from build123d import *

# Parameters (mm, degrees)
SKETCH1_W           = 100
SKETCH1_H           = 58.42
SKETCH1_R           = 2.55
SKETCH1_R_2         = 1.625
SKETCH1_R_3         = 10.5
BOSS_EXTRUDE1_DEPTH = 7.9375
SKETCH2_R           = 4.05
CUT_EXTRUDE1_DEPTH  = 15


with BuildPart() as part:
    # Sketch1 → Boss-Extrude1 (new body)
    with BuildSketch(Plane.XZ.offset(110.068674648)):
        with Locations((45.506748586, 71.609111908)):
            Rectangle(SKETCH1_W, SKETCH1_H)
        with Locations(Location((1.146748586, 95.179111908, 0), (0, 0, 270))):
            Circle(SKETCH1_R, mode=Mode.SUBTRACT)
        with Locations(Location((1.146748586, 48.039111908, 0), (0, 0, 270))):
            Circle(SKETCH1_R, mode=Mode.SUBTRACT)
        with Locations(Location((48.286748586, 48.039111908, 0), (0, 0, 270))):
            Circle(SKETCH1_R, mode=Mode.SUBTRACT)
        with Locations(Location((48.286748586, 95.179111908, 0), (0, 0, 270))):
            Circle(SKETCH1_R, mode=Mode.SUBTRACT)
        with Locations(Location((85.506748586, 85.819111908, 0), (0, 0, 270))):
            Circle(SKETCH1_R_2, mode=Mode.SUBTRACT)
        with Locations(Location((85.506748586, 57.399111908, 0), (0, 0, 270))):
            Circle(SKETCH1_R_2, mode=Mode.SUBTRACT)
        with Locations(Location((24.716748586, 71.609111908, 0), (0, 0, 270))):
            Circle(SKETCH1_R_3, mode=Mode.SUBTRACT)
    extrude(amount=BOSS_EXTRUDE1_DEPTH)

    # Sketch2 → Cut-Extrude1 (cut)
    with BuildSketch(Plane(origin=(95.506748586, -1.5875, 13.918119016), x_dir=(0, 0, -1), z_dir=(1, 0, 0))):
        with Locations((-57.690992892, -108.481174648)):
            Circle(SKETCH2_R)
    extrude(amount=-CUT_EXTRUDE1_DEPTH, mode=Mode.SUBTRACT)


solid = part.part
Verification items for the finished model (mm, model axes). A direction names the side the tool comes from. Round coordinates to 2 decimals unless told otherwise and drop trailing zeros. Write each loop counter-clockwise with the first axis right and the second up, starting at its lowest first coordinate (ties: lowest second). Pieces come first, ordered by that corner, then holes.
(1) Mould release check, pull along Z, two halves, no side actions. Record for faces 1 (the flat face through (80.507, -112, 72)), 2 (the cylindrical face through (84.88, -113.98, 84.32)), 3 (the flat face through (45, -118.006, 72)), 4 (the flat face through (45, -114, 100.819)): pulls with the +Z half, pulls with the -Z half, needs draft (parallel to the pull), parting line crosses it, or undercut.
Returned:
face 1: undercut
face 2: undercut
face 3: needs draft
face 4: pulls with the +Z half
(2) Section check D-D (z = 57.5). Enter the section's corners in (x, y), plus the area to 3 significant figures.
Returned:
outline: (-4.49, -118.01) - (83.88, -118.01) - (83.88, -110.07) - (-4.49, -110.07) - close; (87.13, -118.01) - (95.51, -118.01) - (95.51, -110.07) - (87.13, -110.07) - close
area: 768 mm2
(3) Section check C-C (x = 28.5). Enter the section's corners in (y, z).
Returned:
outline: (-118.01, 42.4) - (-110.07, 42.4) - (-110.07, 61.81) - (-118.01, 61.81) - close; (-118.01, 81.4) - (-110.07, 81.4) - (-110.07, 100.82) - (-118.01, 100.82) - close
(4) Section check B-B (y = -113). Give the number of separate pieces and of enclosed holes in the cut face, plus the area to 3 significant figures.
Returned:
separate pieces: 1
enclosed holes: 7
area: 5,310 mm2
(5) Access from +Z, -Z, +X, -X, +Y, -Y to the whole of each face (thin tool, end or side, straight path). Record for faces 5 (the flat face through (-4.493, -114, 71)), 6 (the cylindrical face through (88.112, -114.118, 71.698)).
Returned:
face 5: +Z, -Z, -X, +Y, -Y
face 6: +X, +Y
(6) Section check A-A (z = 94). Enter the section's corners in (x, y).
Returned:
outline: (-4.49, -118.01) - (-1.11, -118.01) - (-1.11, -110.07) - (-4.49, -110.07) - close; (3.41, -118.01) - (46.03, -118.01) - (46.03, -110.07) - (3.41, -110.07) - close; (50.55, -118.01) - (95.51, -118.01) - (95.51, -110.07) - (50.55, -110.07) - close
(7) Depth check by flat-ended pin: pin 1 Ø2.5 at (x, z) = (85.51, 85.82) entering from -Y; pin 2 Ø3 at (y, z) = (-113, 71) entering from +X. Enter the tip coordinate at first touch or a pass-through.
Returned:
pin 1: passes through
pin 2: stops at x = 95.51
(8) Material ranges on line 1 (X direction, y = -114.75, z = 48); line 2 (X direction, y = -112, z = 49.5); line 3 (Z direction, x = 2, y = -110.25), recorded low to high.
Returned:
line 1: x = -4.49 to -1.4, 3.7 to 45.74, 50.84 to 95.51
line 2: x = -4.49 to -0.94, 3.24 to 46.2, 50.38 to 95.51
line 3: z = 42.4 to 45.64, 50.44 to 92.78, 97.58 to 100.82
